```python
from build123d import *

# Parameters (mm, degrees)
F1_DEPTH = 22
F2_W     = 18
F2_H     = 3
F3_DEPTH = 25
F6_DEPTH = 18
F7_R     = 3
F8_R     = 3
F9_DEPTH = 25


with BuildPart() as f1:
    # F0 (on Front) → F1 (new body)
    with BuildSketch(Plane.XZ):
        with BuildLine():
            ThreePointArc((0, 0), (9, -9), (18, 0))
            Line((18, 0), (18, 18.310677))
            Line((18, 18.310677), (11.310677, 25))
            Line((11.310677, 25), (0, 25))
            Line((0, 25), (0, 0))
        make_face()
    extrude(amount=F1_DEPTH)

    # F2 (on face) → F3 (cut)
    with BuildSketch(Plane(origin=(0, 0, 0), x_dir=(0, -1, 0), z_dir=(-1, 0, 0))):
        with Locations((11, 23.5)):
            Rectangle(F2_W, F2_H)
    extrude(amount=-F3_DEPTH, mode=Mode.SUBTRACT)

    # F5 (on offset) → F6 (cut)
    with BuildSketch(Plane.XZ.offset(2)):
        with BuildLine():
            Line((14.310677, 22), (0, 22))
            ThreePointArc((0, 22), (7.155339, 17.577867), (14.310677, 22))
        make_face()
    extrude(amount=F6_DEPTH, mode=Mode.SUBTRACT)

    # F7
    f7_edges = [f1.edges().sort_by_distance(p)[0] for p in [
        (18, -11, 18.310677),
        (11.310677, -21, 25),
        (11.310677, -1, 25),
        (0, -21, 25),
        (0, -1, 25),
    ]]
    fillet(f7_edges, radius=F7_R)

    # F8 (on face) → F9 (cut)
    with BuildSketch(Plane.XZ.offset(22)):
        with Locations((7.160677, 21.577867)):
            Circle(F8_R)
    extrude(amount=-F9_DEPTH, mode=Mode.SUBTRACT)


solid = f1.part
```
Input: part model. Units: mm. Frame: model coordinates. A direction names the side the tool comes from. Give positions to 0.01 mm unless a question says otherwise; leave off trailing zeros. Order: outer loops, then holes, each group sorted by start corner. A loop starts at its lowest first (then second) coordinate and runs counter-clockwise, first axis right, second up. Notation, with made-up numbers: (-11.5, 45) - (-5.5, 45) arc R14 ccw to (-5.5, 68) - close; hole circle Ø7 at (68, 6.5). An arc over 180 degrees is marked (long way). One line per item, written item: value.
1. Line query: probe 1 along Y at (x, z) = (11.25, 21.5); probe 2 along X at (y, z) = (-11.5, 21); probe 3 along Z at (x, y) = (10, -5.5). Output: solid intervals per line, ascending.
Determined:
probe 1: -22 to -20, -2 to 0
probe 2: 0 to 0.59, 13.72 to 15.31
probe 3: -8.94 to 18.1
2. Reachability of faces 4 (the face through (7.03, -10.87, 17.58)), 5 (the face through (0.86, -1.01, 24.1)) from +Z, -Z, +X, -X, +Y, -Y: full face, straight path, thin tool, end or side. Return the list, or none.
Determined:
face 4: +Z
face 5: +Z, -X, +Y, -Y
3. Cut plane D-D, the plane x = 5.25. Output: boundary loops of the cut face in (y, z) (3 decimals), and give its area (3 significant figures).
Determined:
outline: (-22, -8.182) - (0, -8.182) - (0, 19.265) - (-2, 19.265) - (-2, 17.808) - (-20, 17.808) - (-20, 19.265) - (-22, 19.265) - close; (-22, 23.891) - (-20, 23.891) - (-20, 25) - (-22, 25) - close; (-2, 23.891) - (0, 23.891) - (0, 25) - (-2, 25) - close
area: 582 mm2
4. Pin query (flat end, axial travel): pin 1 Ø2 at (x, y) = (16, -5.5) entering from -Z; pin 2 Ø2 at (x, y) = (8.5, -3.5) entering from +Z; pin 3 Ø3.5 at (x, z) = (7.16, 21.58) entering from -Y. Return the tip coordinate at first contact, or that it passes through.
Determined:
pin 1: z = -6.71
pin 2: z = 17.93
pin 3: through
5. Cut plane C-C, the plane y = -15. Output: boundary loops of the cut face in (x, z).
Determined:
outline: (0, 0) arc R9 ccw to (18, 0) - (18, 17.07) arc R3 ccw to (17.12, 19.19) - (14.31, 22) arc R8 cw to (0, 22) - close
6. Draft query along X for faces 1 (the face through (9, -22, 8)), 2 (the face through (8.77, -21.01, 24.11)), 3 (the face through (17.78, -11.15, 18.2)). Return one class per face: released by +X, released by -X, zero draft, split by the parting line, or undercut.
Determined:
face 1: zero draft
face 2: undercut
face 3: released by +X
7. Cut plane B-B, the plane y = -1.5. Output: boundary loops of the cut face in (x, z), and give its area (3 significant figures).
Determined:
outline: (0, 0) arc R9 ccw to (18, 0) - (18, 17.07) arc R3 ccw to (17.12, 19.19) - (12.19, 24.12) arc R3 ccw to (10.07, 25) - (3, 25) arc R3 ccw to (0, 22) - close; hole circle Ø6 at (7.16, 21.58)
area: 524 mm2
8. Cut plane A-A, the plane x = 9. Output: boundary loops of the cut face in (y, z).
Determined:
outline: (-22, -9) - (0, -9) - (0, 19.21) - (-2, 19.21) - (-2, 17.79) - (-20, 17.79) - (-20, 19.21) - (-22, 19.21) - close; (-22, 23.95) - (-20, 23.95) - (-20, 25) - (-22, 25) - close; (-2, 23.95) - (0, 23.95) - (0, 25) - (-2, 25) - close
